```python
from build123d import *

# Parameters (mm, degrees)
SKETCH_W  = 0.6
SKETCH_H  = 0.65
PAD_DEPTH = 20
FILLET_R  = 0.25


with BuildPart() as part:
    # Sketch → Pad (new body, symmetric)
    with BuildSketch(Plane.XZ):
        Polygon((0.669696, 1.616789), (-0.669696, 1.616789), (-1.616789, 0.669696), (-1.616789, -0.669696), (-0.669696, -1.616789), (0.669696, -1.616789), (1.616789, -0.669696), (1.616789, 0.669696), align=None)
        Rectangle(SKETCH_W, SKETCH_H, mode=Mode.SUBTRACT)
    extrude(amount=PAD_DEPTH, both=True)

    # Fillet
    fillet_edges = [part.edges().sort_by_distance(p)[0] for p in [
        (-1.616789, 0, 0.669696),
        (-1.616789, 0, -0.669696),
        (1.616789, 0, 0.669696),
        (1.616789, 0, -0.669696),
    ]]
    fillet(fillet_edges, radius=FILLET_R)


solid = part.part
```
Can you work these out from the model? Positions are in its coordinate system, mm. Coordinates: 2 decimals unless noted, no trailing zeros. Loops run counter-clockwise (first coordinate to the right, second up) from the corner with the lowest first, then second, coordinate; pieces in that order, holes last.
1) For pin 1 (1.5 mm diameter, centred on y = -10, z = -1, fed in from -X), with a flat end and sliding along its axis, tell me the tip position at first contact or that it passes through.
2) I need wall thicknesses on probe 1 along Z at (x, y) = (-0.05, -10) (3 decimals); probe 2 along X at (y, z) = (2.5, 0); probe 3 along X at (y, z) = (-17.5, 0.6). Which ranges of each line are inside material? Lowest first, please.
3) Imagine slicing it at B-B on x = -1.15. List the corners of the cut face in (y, z) for me.
4) Thinking about a two-plate mould opening in Z: for faces 1 (the flat face through (-1.113, -0.28, -1.174)), 2 (the flat face through (-1.617, 0, 0)), 3 (the flat face through (0, 0, 1.617)), which applies, pulls with the +Z half, pulls with the -Z half, needs draft (parallel to the pull), parting line crosses it, or undercut?
5) Imagine slicing it at A-A on y = 2. List the corners of the cut face in (x, z) for me (3 decimals), plus the area to 3 significant figures.
Completed:
1. pin 1: stops at x = -1.62
2. probe 1: z = -1.617 to -0.325, 0.325 to 1.617
2. probe 2: x = -1.62 to -0.3, 0.3 to 1.62
2. probe 3: x = -1.61 to 1.61
3. outline: (-20, -1.14) - (20, -1.14) - (20, 1.14) - (-20, 1.14) - close
4. face 1: pulls with the -Z half
4. face 2: needs draft
4. face 3: pulls with the +Z half
5. outline: (-1.617, -0.566) arc R0.25 ccw to (-1.544, -0.743) - (-0.67, -1.617) - (0.67, -1.617) - (1.544, -0.743) arc R0.25 ccw to (1.617, -0.566) - (1.617, 0.566) arc R0.25 ccw to (1.544, 0.743) - (0.67, 1.617) - (-0.67, 1.617) - (-1.544, 0.743) arc R0.25 ccw to (-1.617, 0.566) - close; hole (-0.3, -0.325) - (0.3, -0.325) - (0.3, 0.325) - (-0.3, 0.325) - close
5. area: 8.27 mm2
